```python
from build123d import *

# Parameters (mm, degrees)
SKETCH_1_R               = 20.5
EXTRUDE_1_DEPTH          = 7
SKETCH_2_R               = 50
EXTRUDE_2_DEPTH          = 8
CUT_EXTRUDE_1_REACH      = 74.284
SKETCH_3_R               = 16.5
CUT_EXTRUDE_2_REACH      = 73.162
SKETCH_4_R               = 1.6
PATTERN_CIRCULAR_1_COUNT = 6
SKETCH_6_R               = 50
SKETCH_6_R_2             = 27.5
CUT_EXTRUDE_3_DEPTH      = 3
CUT_EXTRUDE_4_REACH      = 74.284
SKETCH_7_R               = 1.6
PATTERN_CIRCULAR_2_COUNT = 8
CUT_EXTRUDE_5_REACH      = 73.414
PATTERN_CIRCULAR_3_COUNT = 8
SKETCH_11_R              = 20.5
EXTRUDE_3_DEPTH          = 4
SKETCH_12_R              = 2.025
CUT_EXTRUDE_6_DEPTH      = 72.561162651
SKETCH_13_R              = 5
CUT_EXTRUDE_7_DEPTH      = 73.284161474
SKETCH_14_R              = 20.5
CUT_EXTRUDE_8_DEPTH      = 73.284161474


with BuildPart() as part:
    # 草图1 → 凸台-拉伸1 (new body)
    with BuildSketch(Plane(origin=(0, 0, 0), x_dir=(1, 0, 0), z_dir=(0, 1, 0))):
        with Locations(Location((0, 0, 0), (0, 0, 270))):
            Circle(SKETCH_1_R)
    extrude(amount=EXTRUDE_1_DEPTH)

    # 草图2 → 凸台-拉伸2 (add)
    with BuildSketch(Plane(origin=(0, 7, 0), x_dir=(1, 0, 0), z_dir=(0, 1, 0))):
        with Locations(Location((0, 0, 0), (0, 0, 270))):
            Circle(SKETCH_2_R)
    extrude(amount=EXTRUDE_2_DEPTH)

    # 草图3 → 切除-拉伸1 (cut, up to next)
    with BuildSketch(Plane.XZ, mode=Mode.PRIVATE) as cut_extrude_1_sk1:
        with Locations(Location((0, 0, 0), (0, 0, 270))):
            Circle(SKETCH_3_R)
    cut_extrude_1_tool1 = extrude(cut_extrude_1_sk1.sketch, amount=-CUT_EXTRUDE_1_REACH, mode=Mode.PRIVATE) & part.part
    add(cut_extrude_1_tool1.solids().sort_by_distance((0, 0, 0))[0], mode=Mode.SUBTRACT)

    # 草图4 → 切除-拉伸2 (cut, up to next)
    with BuildSketch(Plane.XZ.offset(-7), mode=Mode.PRIVATE) as cut_extrude_2_sk1:
        with Locations(Location((0, 24, 0), (0, 0, 270))):
            Circle(SKETCH_4_R)
    cut_extrude_2_tool1 = extrude(cut_extrude_2_sk1.sketch, amount=-CUT_EXTRUDE_2_REACH, mode=Mode.PRIVATE) & part.part
    cut_extrude_2 = cut_extrude_2_tool1.solids().sort_by_distance((0, 7, 24))[0]
    add(cut_extrude_2, mode=Mode.SUBTRACT)

    # 阵列(圆周)1: 切除-拉伸2 ×6 about axis
    pattern_circular_1_axis = Axis((0, 0, 0), (0, 1, 0))
    for i in range(1, PATTERN_CIRCULAR_1_COUNT):
        add(cut_extrude_2.rotate(pattern_circular_1_axis, i * 360 / PATTERN_CIRCULAR_1_COUNT), mode=Mode.SUBTRACT)

    # 草图6 → 切除-拉伸3 (cut)
    with BuildSketch(Plane.XZ.offset(-7)):
        with Locations(Location((0, 0, 0), (0, 0, 270))):
            Circle(SKETCH_6_R)
        with Locations(Location((0, 0, 0), (0, 0, 270))):
            Circle(SKETCH_6_R_2, mode=Mode.SUBTRACT)
    extrude(amount=-CUT_EXTRUDE_3_DEPTH, mode=Mode.SUBTRACT)

    # 草图7 → 切除-拉伸4 (cut, up to next)
    with BuildSketch(Plane(origin=(0, 15, 0), x_dir=(1, 0, 0), z_dir=(0, 1, 0)), mode=Mode.PRIVATE) as cut_extrude_4_sk1:
        with Locations(Location((0, 45, 0), (0, 0, 270))):
            Circle(SKETCH_7_R)
    cut_extrude_4_tool1 = extrude(cut_extrude_4_sk1.sketch, amount=-CUT_EXTRUDE_4_REACH, mode=Mode.PRIVATE) & part.part
    cut_extrude_4 = cut_extrude_4_tool1.solids().sort_by_distance((0, 15, -45))[0]
    add(cut_extrude_4, mode=Mode.SUBTRACT)

    # 阵列(圆周)2: 切除-拉伸4 ×8 about axis
    pattern_circular_2_axis = Axis((0, 0, 0), (0, 1, 0))
    for i in range(1, PATTERN_CIRCULAR_2_COUNT):
        add(cut_extrude_4.rotate(pattern_circular_2_axis, i * 360 / PATTERN_CIRCULAR_2_COUNT), mode=Mode.SUBTRACT)

    # 草图9 → 切除-拉伸5 (cut, up to next)
    with BuildSketch(Plane.XZ.offset(-10), mode=Mode.PRIVATE) as cut_extrude_5_sk1:
        with BuildLine():
            ThreePointArc((-7.46687164, 42.34673338), (-16.455387592, 39.726819898), (-24.663786763, 35.223537904))
            ThreePointArc((-24.663786763, 35.223537904), (-27.449243724, 35.71468912), (-26.958092508, 38.500146082))
            ThreePointArc((-26.958092508, 38.500146082), (-17.986121321, 43.422338028), (-8.16146435, 46.285964392))
            ThreePointArc((-8.16146435, 46.285964392), (-5.844552489, 44.663645241), (-7.46687164, 42.34673338))
        make_face()
    cut_extrude_5_tool1 = extrude(cut_extrude_5_sk1.sketch, amount=-CUT_EXTRUDE_5_REACH, mode=Mode.PRIVATE) & part.part
    cut_extrude_5 = cut_extrude_5_tool1.solids().sort_by_distance((-17.046965, 10, 41.155015))[0]
    add(cut_extrude_5, mode=Mode.SUBTRACT)

    # 阵列(圆周)3: 切除-拉伸5 ×8 about axis
    pattern_circular_3_axis = Axis((0, 0, 0), (0, 1, 0))
    for i in range(1, PATTERN_CIRCULAR_3_COUNT):
        add(cut_extrude_5.rotate(pattern_circular_3_axis, i * 360 / PATTERN_CIRCULAR_3_COUNT), mode=Mode.SUBTRACT)

    # 草图11 → 凸台-拉伸3 (add)
    with BuildSketch(Plane.XZ):
        with Locations(Location((0, 0, 0), (0, 0, 90))):
            Circle(SKETCH_11_R)
    extrude(amount=-EXTRUDE_3_DEPTH)

    # 草图12 → 切除-拉伸6 (cut, through all)
    with BuildSketch(Plane(origin=(0, 4, 0), x_dir=(1, 0, 0), z_dir=(0, 1, 0))):
        with Locations(Location((0, 11.5, 0), (0, 0, 270))):
            Circle(SKETCH_12_R)
        with Locations(Location((11.5, 0, 0), (0, 0, 270))):
            Circle(SKETCH_12_R)
        with Locations(Location((0, -11.5, 0), (0, 0, 270))):
            Circle(SKETCH_12_R)
        with Locations(Location((-11.5, 0, 0), (0, 0, 270))):
            Circle(SKETCH_12_R)
    extrude(amount=-CUT_EXTRUDE_6_DEPTH, mode=Mode.SUBTRACT)

    # 草图13 → 切除-拉伸7 (cut, through all)
    with BuildSketch(Plane.XZ):
        with Locations(Location((0, 0, 0), (0, 0, 270))):
            Circle(SKETCH_13_R)
    extrude(amount=-CUT_EXTRUDE_7_DEPTH, mode=Mode.SUBTRACT)

    # 草图14 → 切除-拉伸8 (cut, through all)
    with BuildSketch(Plane.XZ):
        with Locations(Location((0, 0, 0), (0, 0, 270))):
            Circle(SKETCH_14_R)
    extrude(amount=-CUT_EXTRUDE_8_DEPTH, mode=Mode.SUBTRACT)


solid = part.part
```
The listing builds one solid part. Answer for the finished solid, in the listing's coordinates (mm). Round coordinates to 2 decimals unless told otherwise and drop trailing zeros. Order: outer loops, then holes, each group sorted by start corner. A loop starts at its lowest first (then second) coordinate and runs counter-clockwise, first axis right, second up. Notation, with made-up numbers: (-28, -7.75) -> (8, -7.75) arc R25 ccw to (8, 29.25) -> close; hole circle Ø1 at (73.5, 88). An arc over 180 degrees is marked (long way). Answer as CSV lines item,"result".
Q1. Given pin 1 (1.9 mm diameter, centred on x = -20.78, z = 12, fed in from +Y); pin 2 (1 mm diameter, centred on x = 8.5, y = 10, fed in from +Z); pin 3 (6 mm diameter, centred on x = 39, z = 5, fed in from -Y); pin 4 (2 mm diameter, centred on x = -6, z = 19, fed in from +Y), each flat-ended and moving along its own axis, determine where each tip first touches the part or whether it passes through.
Computed values:
pin 1,"passes through"
pin 2,"stops at z = 49.36"
pin 3,"stops at y = 10"
pin 4,"stops at y = 15"
Q2. A cutting plane is placed at A-A on x = 0. Determine the outline of the cut face in (y, z).
Computed values:
outline,"(7, -27.5) -> (10, -27.5) -> (10, -43.4) -> (15, -43.4) -> (15, -25.6) -> (7, -25.6) -> close; (7, -22.4) -> (15, -22.4) -> (15, -20.5) -> (7, -20.5) -> close; (7, 20.5) -> (15, 20.5) -> (15, 22.4) -> (7, 22.4) -> close; (7, 25.6) -> (15, 25.6) -> (15, 43.4) -> (10, 43.4) -> (10, 27.5) -> (7, 27.5) -> close; (10, -50) -> (15, -50) -> (15, -46.6) -> (10, -46.6) -> close; (10, 46.6) -> (15, 46.6) -> (15, 50) -> (10, 50) -> close"
Q3. A cutting plane is placed at D-D on x = 45. Determine the outline of the cut face in (y, z).
Computed values:
outline,"(10, -21.79) -> (15, -21.79) -> (15, -13.56) -> (10, -13.56) -> close; (10, -5.93) -> (15, -5.93) -> (15, -1.6) -> (10, -1.6) -> close; (10, 1.6) -> (15, 1.6) -> (15, 5.93) -> (10, 5.93) -> close; (10, 13.56) -> (15, 13.56) -> (15, 21.79) -> (10, 21.79) -> close"
Q4. A cutting plane is placed at C-C on y = 8.5. Determine the outline of the cut face in (x, z).
Computed values:
outline,"circle Ø55 at (0, 0); hole circle Ø3.2 at (-20.78, -12); hole circle Ø3.2 at (-20.78, 12); hole circle Ø41 at (0, 0); hole circle Ø3.2 at (0, -24); hole circle Ø3.2 at (0, 24); hole circle Ø3.2 at (20.78, -12); hole circle Ø3.2 at (20.78, 12)"
Q5. For a pull along Z with two mould halves and no side action, classify faces 1 (the cylindrical face through (27.474, 12.465, 35.751)), 2 (the cylindrical face through (39.78, 12.46, 16.33)) as +Z half, -Z half, draft (parallel to the pull), parting line (faces both ways), or undercut.
Computed values:
face 1,"undercut"
face 2,"undercut"
Q6. Consider line 1 (Z direction, x = 24.5, y = 10.5); line 2 (X direction, y = 8, z = -11); line 3 (Y direction, x = -23, z = 27). Determine where each line is inside the solid, lowest interval first. Write a range as from..to.
Computed values:
line 1,"z = -43.59..-40.11, -35.34..35.34, 40.11..43.59"
line 2,"x = -25.2..-22.03, -19.54..-17.3, 17.3..19.54, 22.03..25.2"
line 3,"y = 10..15"
Q7. A cutting plane is placed at B-B on z = 0. Determine the outline of the cut face in (x, y).
Computed values:
outline,"(-50, 10) -> (-46.6, 10) -> (-46.6, 15) -> (-50, 15) -> close; (-43.4, 10) -> (-27.5, 10) -> (-27.5, 7) -> (-20.5, 7) -> (-20.5, 15) -> (-43.4, 15) -> close; (20.5, 7) -> (27.5, 7) -> (27.5, 10) -> (43.4, 10) -> (43.4, 15) -> (20.5, 15) -> close; (46.6, 10) -> (50, 10) -> (50, 15) -> (46.6, 15) -> close"
